Autodesk Inventor part; units mm, degrees
ref_plane "Начальная плоскость" through (0, 0, 319.5) normal (0, 0, 1) x (1, 0, 0)
ref_plane "Конечная плоскость" through (0, 0, 667) normal (0, 0, 1) x (1, 0, 0)
ref_plane "РабПлоскость8" through (0, 32.5, 319.5) normal (0, 0, -1) x (-1, 0, 0)
ref_plane "Начальная плоскость" through (0, 0, 319.5) normal (0, 0, 1) x (1, 0, 0)
ref_plane "Конечная плоскость" through (0, 0, 667) normal (0, 0, 1) x (1, 0, 0)
sketch "Эскиз" plane through (0, 0, 0) normal (0, 0, 1) x (1, 0, 0)
  line L0 (36, -32.5) -> (0, -32.5)
  line L1 (36, -32.5) -> (36, -28.696)
  line L2 (33.6994, -26.2039) -> (9.9215, -24.3017)
  line L3 (4.4, -18.3208) -> (4.4, 18.3208)
  line L4 (33.6994, 26.2039) -> (9.9215, 24.3017)
  line L5 (36, 28.696) -> (36, 32.5)
  line L6 (0, 32.5) -> (36, 32.5)
  line L7 (0, -32.5) -> (0, 32.5)
  arc A0 (4.4, -18.3208) -> (9.9215, -24.3017) centre (10.4, -18.3208) ccw
  arc A1 (9.9215, 24.3017) -> (4.4, 18.3208) centre (10.4, 18.3208) ccw
  arc A2 (36, -28.696) -> (33.6994, -26.2039) centre (33.5, -28.696) ccw
  arc A3 (33.6994, 26.2039) -> (36, 28.696) centre (33.5, 28.696) ccw
  line L8 (0, 45.5) -> (0, -45.5) construction
  line L9 (-7.2974, 0) -> (43.7847, 0) construction
  point P0 (36, -26.388)
  point P1 (4.4, -23.86)
  point P2 (4.4, 23.86)
  point P3 (36, 26.388)
  dimension "d3" = 36
  dimension "d5" = 4.4
  dimension "d7" = 65
  dimension "d9" = 8.64
  dimension "d11" = 8.64
  dimension "d13" = 6.112
  dimension "d15" = 6.112
  dimension "d22" = 6
  dimension "d23" = 2.5
  dimension "d24" = 32.5
  dimension "d25" = 0
extrude "Тело" add sketch "Эскиз" along normal up to surface (347.5 mm away) from surface at 319.5
sketch "Sketch3" plane through (0, 0, 0) normal (0, 0, 1) x (1, 0, 0)
  line L0 (0, 0) -> (10, 0)
ref_plane "Work Plane7" through (0, 0, 0) normal (0, -1, 0) x (1, 0, 0)
sketch "Sketch4" plane through (0, 0, 0) normal (0, -1, 0) x (1, 0, 0)
  line L0 (-2, 319.5) -> (12, 319.5)
  line L1 (-2, 667) -> (12, 667)
  dimension "d29" = 347.5
ref_plane "РабПлоскость8" through (0, 32.5, 319.5) normal (0, 0, -1) x (-1, 0, 0)
split "Разделение1" plane through (0, 32.5, 319.5) removes the side toward (0, 0, -1)
equation "\"d3\" = b"
equation "\"d7\" = ParH"
equation "\"d22\" = R"
equation "\"d23\" = R1"
equation "\"d24\" = 0.5 * d7"
equation "\"d16\" = G_L"
equation "\"R1\" = 2.5"
equation "\"R\" = 6"
equation "\"t1\" = 4.4"
equation "\"t2\" = 7.2"
equation "\"ParH\" = 65"
equation "\"b\" = 36"
equation "\"msp_x1\" = 0.04 * b"
equation "\"msp_x2\" = -0.08 * t1 + 0.04 * b"
equation "\"G_L\" = d29"
equation "\"ex\" = 0"
equation "\"G_OFFSET_START\" = -319.5"
equation "\"G_OFFSET_END\" = 0"
equation "\"d26\" = -G_OFFSET_START"
equation "\"d27\" = G_OFFSET_END + B_L"
equation "\"B_L\" = 667"
properties part number "Швеллер 6.5U-347,5 ГОСТ 8240-97" material "Сталь, мягкая"
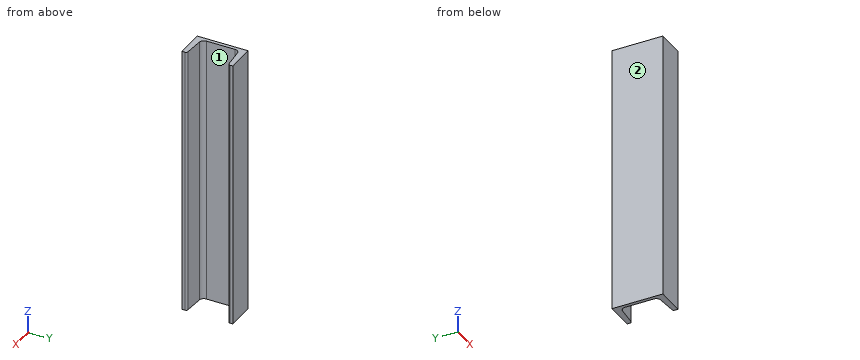
Build history of the part. All positions in model axes, mm. Face numbers are marked on the shaded views. Round coordinates to 2 decimals unless told otherwise and drop trailing zeros. Write each loop counter-clockwise with the first axis right and the second up, starting at its lowest first coordinate (ties: lowest second). Pieces come first, ordered by that corner, then holes. Notation, with made-up numbers: M -26,85.25 L -11,85.25 A27 ccw -11,103.25 Z; hole C 67,35 d1. An arc over 180 degrees is marked long. Answer in a Markdown table with one row per item.
1. Saw through at C-C (y = -4). List the corners of the cut face in (x, z), and give its area (3 significant figures).
Geometry check:
| item | result |
|---|---|
| outline | M 0,319.5 L 4.4,319.5 L 4.4,667 L 0,667 Z |
| area | 1,530 mm2 |
2. Saw through at B-B (z = 389.5). List the corners of the cut face in (x, y).
Geometry check:
| item | result |
|---|---|
| outline | M 0,-32.5 L 36,-32.5 L 36,-28.7 A2.5 ccw 33.7,-26.2 L 9.92,-24.3 A6 cw 4.4,-18.32 L 4.4,18.32 A6 cw 9.92,24.3 L 33.7,26.2 A2.5 ccw 36,28.7 L 36,32.5 L 0,32.5 Z |
3. Mould opens along Y. For the marked faces 1 and 2 say: +Y half, -Y half, draft (parallel to the pull), parting line (faces both ways), or undercut.
Geometry check:
| item | result |
|---|---|
| face 1 | undercut |
| face 2 | draft |
4. Probe L1, parallel to Y at x = 33, z = 543; L2, parallel to X at y = 2, z = 513.5; L3, parallel to Y at x = 10, z = 356.5. List the from-to ranges inside material, lowest first. Write a range as [from, to].
Geometry check:
| item | result |
|---|---|
| L1 | [-32.5, -26.15], [26.15, 32.5] |
| L2 | [0, 4.4] |
| L3 | [-32.5, -24.31], [24.31, 32.5] |
5. Saw through at A-A (x = 26.5). List the corners of the cut face in (y, z).
Geometry check:
| item | result |
|---|---|
| outline | M -32.5,319.5 L -25.63,319.5 L -25.63,667 L -32.5,667 Z; M 25.63,319.5 L 32.5,319.5 L 32.5,667 L 25.63,667 Z |
6. Flat gauge pins, fed straight in: P1, Ø2, axis at y = -6.5, z = 574.5, coming from the -X side; P2, Ø18.5, axis at y = 0, z = 438, coming from the +X side. Where does each tip first touch, or does it go through?
Geometry check:
| item | result |
|---|---|
| P1 | x = 0 |
| P2 | x = 4.4 |
